from build123d import *

# Parameters (mm, degrees)
F0_W     = 60
F0_H     = 40
F1_DEPTH = 40
F2_W     = 20
F2_H     = 20
F3_DEPTH = 40.001
F5_DEPTH = 40.001


with BuildPart() as f1:
    # F0 (on Front) → F1 (new body)
    with BuildSketch(Plane.XZ):
        with Locations((30, 20)):
            Rectangle(F0_W, F0_H)
    extrude(amount=-F1_DEPTH)

    # F2 (on face) → F3 (cut, through all)
    with BuildSketch(Plane.XZ):
        with Locations((50, 30)):
            Rectangle(F2_W, F2_H)
    extrude(amount=-F3_DEPTH, mode=Mode.SUBTRACT)

    # F4 (on face) → F5 (cut, through all)
    with BuildSketch(Plane.XY.offset(40)):
        Polygon((20, 0), (0, 20), (0, 0), align=None)
    extrude(amount=-F5_DEPTH, mode=Mode.SUBTRACT)


solid = f1.part
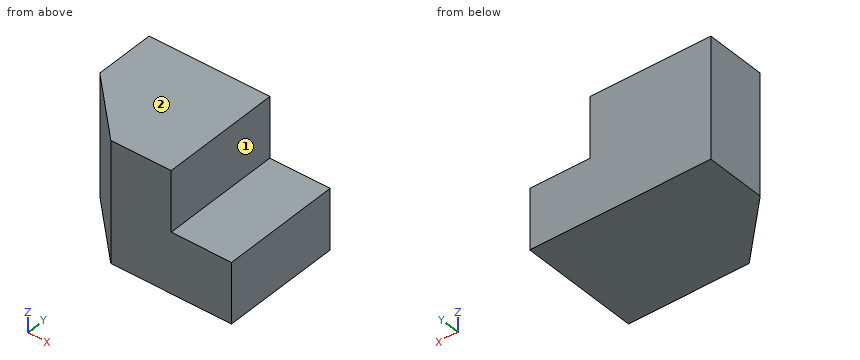
Input: part model. Units: mm. Frame: model coordinates. Face numbers are marked on the shaded views. A direction names the side the tool comes from. Coordinates: 2 decimals unless noted, no trailing zeros. Order: outer loops, then holes, each group sorted by start corner. A loop starts at its lowest first (then second) coordinate and runs counter-clockwise, first axis right, second up.
1. Ray query, line 1 along X through (y, z) = (28, 29); line 2 along Z through (x, y) = (40.5, 4); line 3 along Y through (x, z) = (19, 26). Return the intervals inside material, ascending.
Checked values:
line 1: x = 0 to 40
line 2: z = 0 to 20
line 3: y = 1 to 40
2. Access query for the marked faces 1 and 2. Directions: +Z, -Z, +X, -X, +Y, -Y. A direction counts if a zero-diameter tool reaches every point of the face in a straight line with its end or side. Return the directions, or none.
Checked values:
face 1: +Z, +X, +Y, -Y
face 2: +Z, +X, -X, +Y, -Y
3. Cut plane B-B, the plane z = 13. Return loops of the section in (x, y), plus the area to 3 significant figures.
Checked values:
outline: (0, 20) - (20, 0) - (60, 0) - (60, 40) - (0, 40) - close
area: 2,200 mm2
4. Cut plane D-D, the plane y = 5. Return loops of the section in (x, z).
Checked values:
outline: (15, 0) - (60, 0) - (60, 20) - (40, 20) - (40, 40) - (15, 40) - close
5. Contact query for flat-ended pins moving along their axis: P1, Ø2, axis at y = 15, z = 27, coming from the +X side; P2, Ø1.5, axis at x = 13, z = 19, coming from the -Y side; P3, Ø22, axis at x = 54, y = 20.5, coming from the +Z side. Output: stop coordinate, or through.
Checked values:
P1: stops at x = 40
P2: stops at y = 6.25
P3: stops at z = 20
6. Cut plane C-C, the plane x = 51. Return loops of the section in (y, z), plus the area to 3 significant figures.
Checked values:
outline: (0, 0) - (40, 0) - (40, 20) - (0, 20) - close
area: 800 mm2
7. Cut plane A-A, the plane y = 25.5. Return loops of the section in (x, z), plus the area to 3 significant figures.
Checked values:
outline: (0, 0) - (60, 0) - (60, 20) - (40, 20) - (40, 40) - (0, 40) - close
area: 2,000 mm2
